```python
from build123d import *

# Parameters (mm, degrees)
F0_W     = 35
F0_H     = 35
F0_W_2   = 31
F0_H_2   = 31
F1_DEPTH = 4
F0_W_3   = 2.1
F0_H_3   = 16
F0_W_4   = 2.1574016428
F0_H_4   = 6.115043208
F2_DEPTH = 2
F4_D     = 4


with BuildPart() as f1:
    # F0 (on Top) → F1 (new body)
    with BuildSketch(Plane.XY):
        with Locations((5.448846221, -1.0115454492)):
            Rectangle(F0_W, F0_H)
        with Locations((5.448846221, -1.0115454492)):
            Rectangle(F0_W_2, F0_H_2, mode=Mode.SUBTRACT)
    extrude(amount=F1_DEPTH)



with BuildPart() as f1b:
    # F0 (on Top) → F1, piece 2 (new body)
    with BuildSketch(Plane.XY):
        with BuildLine():
            Line((1.8578098388, -0.9776405059), (4.0152114816, -0.9776405059))
            Line((4.0152114816, -0.9776405059), (4.0418037977, -0.9776405059))
            ThreePointArc((4.0418037977, -0.9776405059), (6.1631241413, -0.0989608494), (7.0418037977, 2.0223594941))
            Line((7.0418037977, 2.0223594941), (7.0418037977, 5.4223594941))
            Line((7.0418037977, 5.4223594941), (3.9449525066, 5.4223594941))
            Line((3.9449525066, 5.4223594941), (2.7918037977, 5.4223594941))
            Line((2.7918037977, 5.4223594941), (1.6386550888, 5.4223594941))
            Line((1.6386550888, 5.4223594941), (-1.4581962023, 5.4223594941))
            Line((-1.4581962023, 5.4223594941), (-1.4581962023, 2.0223594941))
            ThreePointArc((-1.4581962023, 2.0223594941), (-0.5795165459, -0.0989608494), (1.5418037977, -0.9776405059))
            Line((1.5418037977, -0.9776405059), (1.8578098388, -0.9776405059))
        make_face()
        with BuildLine():
            ThreePointArc((0.3418037977, 6.9223594941), (1.3332450808, 6.4689196757), (1.6386550888, 5.4223594941))
            Line((1.6386550888, 5.4223594941), (2.7918037977, 5.4223594941))
            Line((2.7918037977, 5.4223594941), (2.7918037977, 7.8223594941))
            ThreePointArc((2.7918037977, 7.8223594941), (1.7058510843, 8.7062477042), (0.3418037977, 9.0223594941))
            Line((0.3418037977, 9.0223594941), (-1.4581962023, 9.0223594941))
            Line((-1.4581962023, 9.0223594941), (-1.4581962023, 6.9223594941))
            Line((-1.4581962023, 6.9223594941), (0.3418037977, 6.9223594941))
        make_face()
        with BuildLine():
            Line((2.7918037977, 5.4223594941), (3.9449525066, 5.4223594941))
            ThreePointArc((3.9449525066, 5.4223594941), (4.2503625146, 6.4689196757), (5.2418037977, 6.9223594941))
            Line((5.2418037977, 6.9223594941), (7.0418037977, 6.9223594941))
            Line((7.0418037977, 6.9223594941), (7.0418037977, 9.0223594941))
            Line((7.0418037977, 9.0223594941), (5.2418037977, 9.0223594941))
            ThreePointArc((5.2418037977, 9.0223594941), (3.8777565111, 8.7062477042), (2.7918037977, 7.8223594941))
            Line((2.7918037977, 7.8223594941), (2.7918037977, 5.4223594941))
        make_face()
        with Locations((10.0591945603, 0.9073162861)):
            Rectangle(F0_W_3, F0_H_3)
        with BuildLine():
            Line((11.1091945603, -7.0926837139), (9.0091945603, -7.0926837139))
            ThreePointArc((9.0091945603, -7.0926837139), (6.512203021, -9.5896752533), (4.0152114816, -7.0926837139))
            Line((4.0152114816, -7.0926837139), (1.8578098388, -7.0926837139))
            ThreePointArc((1.8578098388, -7.0926837139), (6.4835021996, -11.7183760746), (11.1091945603, -7.0926837139))
        make_face()
        with Locations((2.9365106602, -4.0351621099)):
            Rectangle(F0_W_4, F0_H_4)
    extrude(amount=F1_DEPTH)


with BuildPart() as f1_1:
    add(f1.part)

    add(f1b.part)  # F2 merges F1b
    # F0 (on Top) → F2 (join)
    with BuildSketch(Plane.XY):
        with Locations((5.448846221, -1.0115454492)):
            Rectangle(F0_W_2, F0_H_2)
        with BuildLine():
            Line((9.0091945603, -7.0926837139), (9.0091945603, 8.9073162861))
            Line((9.0091945603, 8.9073162861), (11.1091945603, 8.9073162861))
            Line((11.1091945603, 8.9073162861), (11.1091945603, -7.0926837139))
            ThreePointArc((11.1091945603, -7.0926837139), (6.4835021996, -11.7183760746), (1.8578098388, -7.0926837139))
            Line((1.8578098388, -7.0926837139), (1.8578098388, -0.9776405059))
            Line((1.8578098388, -0.9776405059), (1.5418037977, -0.9776405059))
            ThreePointArc((1.5418037977, -0.9776405059), (-0.5795165459, -0.0989608494), (-1.4581962023, 2.0223594941))
            Line((-1.4581962023, 2.0223594941), (-1.4581962023, 5.4223594941))
            Line((-1.4581962023, 5.4223594941), (1.6386550888, 5.4223594941))
            ThreePointArc((1.6386550888, 5.4223594941), (1.3332450808, 6.4689196757), (0.3418037977, 6.9223594941))
            Line((0.3418037977, 6.9223594941), (-1.4581962023, 6.9223594941))
            Line((-1.4581962023, 6.9223594941), (-1.4581962023, 9.0223594941))
            Line((-1.4581962023, 9.0223594941), (0.3418037977, 9.0223594941))
            ThreePointArc((0.3418037977, 9.0223594941), (1.7058510843, 8.7062477042), (2.7918037977, 7.8223594941))
            ThreePointArc((2.7918037977, 7.8223594941), (3.8777565111, 8.7062477042), (5.2418037977, 9.0223594941))
            Line((5.2418037977, 9.0223594941), (7.0418037977, 9.0223594941))
            Line((7.0418037977, 9.0223594941), (7.0418037977, 6.9223594941))
            Line((7.0418037977, 6.9223594941), (5.2418037977, 6.9223594941))
            ThreePointArc((5.2418037977, 6.9223594941), (4.2503625146, 6.4689196757), (3.9449525066, 5.4223594941))
            Line((3.9449525066, 5.4223594941), (7.0418037977, 5.4223594941))
            Line((7.0418037977, 5.4223594941), (7.0418037977, 2.0223594941))
            ThreePointArc((7.0418037977, 2.0223594941), (6.1631241413, -0.0989608494), (4.0418037977, -0.9776405059))
            Line((4.0418037977, -0.9776405059), (4.0152114816, -0.9776405059))
            Line((4.0152114816, -0.9776405059), (4.0152114816, -7.0926837139))
            ThreePointArc((4.0152114816, -7.0926837139), (6.512203021, -9.5896752533), (9.0091945603, -7.0926837139))
        make_face(mode=Mode.SUBTRACT)
    extrude(amount=F2_DEPTH)

    # F4 (through all)
    with Locations(Plane.XY.offset(2)):
        with Locations((17.948846221, 11.4884545508)):
            Hole(F4_D / 2)


solid = f1_1.part
```
Geometry: final body of the model. Coordinates: model frame, mm. A direction names the side the tool comes from. Round coordinates to 2 decimals unless told otherwise and drop trailing zeros. Write each loop counter-clockwise with the first axis right and the second up, starting at its lowest first coordinate (ties: lowest second). Pieces come first, ordered by that corner, then holes. Notation, with made-up numbers: (69, 61) -> (73, 61) arc R29 ccw to (73, 84) -> close; hole circle Ø6 at (34, 59). An arc over 180 degrees is marked (long way). Use CSV: the item, a comma, the result in double quotes. Start each with the question number.
Q1. Line query: L1, parallel to X at y = -0.5, z = 2.4; L2, parallel to Y at x = 15, z = 2.4; L3, parallel to X at y = 10, z = 3.15. Output: solid intervals per line, ascending.
Q2. Section C-C (y = -4.5). Return loops of the section in (x, z), plus the area to 3 significant figures.
Q3. Pull-direction query (X, two-part tool) for faces 3 (the face through (5, -18.512, 2)), 4 (the face through (6.14, -0.12, 2.99)), 5 (the face through (6.382, -11.717, 2.986)), 6 (the face through (-12.051, -1, 2)); classes: pulls with the +X half, pulls with the -X half, needs draft (parallel to the pull), parting line crosses it, or undercut.
Q4. Section B-B (x = 15). Return loops of the section in (y, z), plus the area to 3 significant figures.
Q5. Reachability of faces 1 (the face through (5, 14.488, 3)), 2 (the face through (5, 1, 4)) from +Z, -Z, +X, -X, +Y, -Y: full face, straight path, thin tool, end or side. Return the list, or none.
Q6. Section A-A (y = -13.5). Return loops of the section in (x, z).
Q7. Section D-D (x = 10.5). Return loops of the section in (y, z).
Result sheet:
1,L1,"-12.05 to -10.05, -0.08 to 5.67, 9.01 to 11.11, 20.95 to 22.95"
1,L2,"-18.51 to -16.51, 14.49 to 16.49"
1,L3,"-12.05 to -10.05, 20.95 to 22.95"
2,outline,"(-12.05, 0) -> (22.95, 0) -> (22.95, 4) -> (20.95, 4) -> (20.95, 2) -> (11.11, 2) -> (11.11, 4) -> (9.01, 4) -> (9.01, 2) -> (4.02, 2) -> (4.02, 4) -> (1.86, 4) -> (1.86, 2) -> (-10.05, 2) -> (-10.05, 4) -> (-12.05, 4) -> close"
2,area,"86.5 mm²"
3,face 3,"needs draft"
3,face 4,"undercut"
3,face 5,"undercut"
3,face 6,"pulls with the -X half"
4,outline,"(-18.51, 0) -> (16.49, 0) -> (16.49, 4) -> (14.49, 4) -> (14.49, 2) -> (-16.51, 2) -> (-16.51, 4) -> (-18.51, 4) -> close"
4,area,"78.0 mm²"
5,face 1,"+Z"
5,face 2,"+Z, +X, -X, +Y, -Y"
6,outline,"(-12.05, 0) -> (22.95, 0) -> (22.95, 4) -> (20.95, 4) -> (20.95, 2) -> (-10.05, 2) -> (-10.05, 4) -> (-12.05, 4) -> close"
7,outline,"(-18.51, 0) -> (16.49, 0) -> (16.49, 4) -> (14.49, 4) -> (14.49, 2) -> (8.91, 2) -> (8.91, 4) -> (-9.39, 4) -> (-9.39, 2) -> (-16.51, 2) -> (-16.51, 4) -> (-18.51, 4) -> close"
